Input: part model. Units: mm. Frame: model coordinates. Round coordinates to 2 decimals unless told otherwise and drop trailing zeros. Loops run counter-clockwise (first coordinate to the right, second up) from the corner with the lowest first, then second, coordinate; pieces in that order, holes last.
(1) Cut plane A-A, the plane z = 19.8. Output: boundary loops of the cut face in (x, y).
(2) First-contact query: pin 1 Ø1.6 at (x, z) = (0, 5.8) entering from +Y; pin 2 Ø2.5 at (x, z) = (7, 12.8) entering from -Y; pin 3 Ø3 at (x, z) = (-7, 12.8) entering from +Y; pin 4 Ø5.5 at (x, z) = (0, 5.8) entering from -Y. Flat tips, straight axial feed; report the tip coordinate or a pass-through.
(3) Cut plane B-B, the plane x = 0. Output: boundary loops of the cut face in (y, z).
(4) Line query: line 1 (Z direction, x = 0, y = 1.6); line 2 (Z direction, x = 7, y = 2.3); line 3 (Z direction, x = 0, y = 0.9). Output: solid intervals per line, ascending.
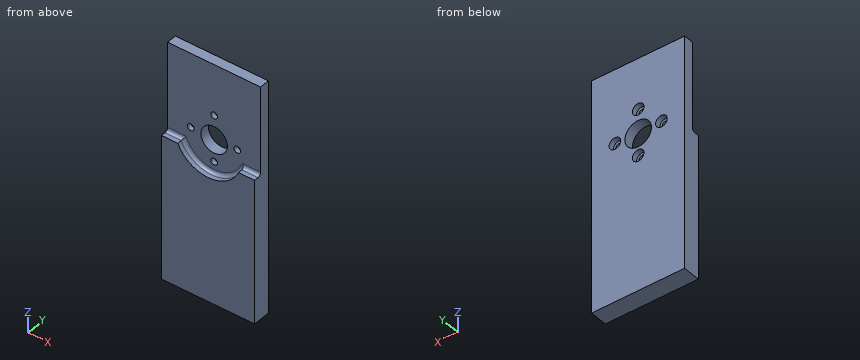
from build123d import *

# Parameters (mm, degrees)
SKETCH1_W           = 28
SKETCH1_H           = 70.4
BOSS_EXTRUDE1_DEPTH = 3
SKETCH4_R           = 1
CUT_EXTRUDE2_DEPTH  = 10
SKETCH5_R           = 4
CUT_EXTRUDE3_DEPTH  = 10
SKETCH10_R          = 1.75
CUT_EXTRUDE9_DEPTH  = 1.6
BOSS_EXTRUDE2_DEPTH = 2.3
FILLET1_R           = 1


with BuildPart() as part:
    # Sketch1 → Boss-Extrude1 (new body)
    with BuildSketch(Plane(origin=(0, 0, 0), x_dir=(1, 0, 0), z_dir=(0, 1, 0))):
        Rectangle(SKETCH1_W, SKETCH1_H)
    extrude(amount=BOSS_EXTRUDE1_DEPTH)

    # Sketch4 → Cut-Extrude2 (cut)
    with BuildSketch(Plane(origin=(0, 3, 0), x_dir=(1, 0, 0), z_dir=(0, 1, 0))):
        with Locations((7, -12.8)):
            Circle(SKETCH4_R)
        with Locations((0, -19.8)):
            Circle(SKETCH4_R)
        with Locations((-7, -12.8)):
            Circle(SKETCH4_R)
        with Locations((0, -5.8)):
            Circle(SKETCH4_R)
    extrude(amount=-CUT_EXTRUDE2_DEPTH, mode=Mode.SUBTRACT)

    # Sketch5 → Cut-Extrude3 (cut)
    with BuildSketch(Plane(origin=(0, 3, 0), x_dir=(1, 0, 0), z_dir=(0, 1, 0))):
        with Locations((0, -12.4)):
            Circle(SKETCH5_R)
    extrude(amount=-CUT_EXTRUDE3_DEPTH, mode=Mode.SUBTRACT)

    # Sketch10 → Cut-Extrude9 (cut)
    with BuildSketch(Plane(origin=(0, 3, 0), x_dir=(1, 0, 0), z_dir=(0, 1, 0))):
        with Locations((0, -19.8)):
            Circle(SKETCH10_R)
        with Locations((-7, -12.8)):
            Circle(SKETCH10_R)
        with Locations((0, -5.8)):
            Circle(SKETCH10_R)
        with Locations((7, -12.8)):
            Circle(SKETCH10_R)
    extrude(amount=-CUT_EXTRUDE9_DEPTH, mode=Mode.SUBTRACT)

    # Sketch11 → Boss-Extrude2 (add)
    with BuildSketch(Plane.XZ):
        with BuildLine():
            Line((9.143433638, 8.350602353), (14, 8.350602353))
            Line((14, 8.350602353), (14, -35.2))
            Line((14, -35.2), (-14, -35.2))
            Line((-14, -35.2), (-14, 8.350602353))
            Line((-14, 8.350602353), (-9.143433638, 8.350602353))
            ThreePointArc((-9.143433638, 8.350602353), (0, 2.4), (9.143433638, 8.350602353))
        make_face()
    extrude(amount=BOSS_EXTRUDE2_DEPTH)

    # Fillet1
    fillet1_edges = [part.edges().sort_by_distance(p)[0] for p in [
        (11.571716819, 0, 8.350602353),
        (0, 0, 2.4),
        (-11.571716819, 0, 8.350602353),
    ]]
    fillet(fillet1_edges, radius=FILLET1_R)


solid = part.part
Reported:
1. outline: (-14, 0) - (-1, 0) - (-1, 1.4) - (-1.75, 1.4) - (-1.75, 3) - (-14, 3) - close; (1, 0) - (14, 0) - (14, 3) - (1.75, 3) - (1.75, 1.4) - (1, 1.4) - close
2. pin 1: passes through
2. pin 2: stops at y = 0
2. pin 3: stops at y = 1.4
2. pin 4: stops at y = -0.06
3. outline: (-2.3, -35.2) - (3, -35.2) - (3, 4.05) - (1.4, 4.05) - (1.4, 4.8) - (0, 4.8) - (0, 3.4) arc R1 cw to (-1, 2.4) - (-2.3, 2.4) - close; (0, 6.8) - (1.4, 6.8) - (1.4, 7.55) - (3, 7.55) - (3, 8.4) - (0, 8.4) - close; (0, 16.4) - (3, 16.4) - (3, 18.05) - (1.4, 18.05) - (1.4, 18.8) - (0, 18.8) - close; (0, 20.8) - (1.4, 20.8) - (1.4, 21.55) - (3, 21.55) - (3, 35.2) - (0, 35.2) - close
4. line 1: z = -35.2 to 4.05, 7.55 to 8.4, 16.4 to 18.05, 21.55 to 35.2
4. line 2: z = -35.2 to 11.05, 14.55 to 35.2
4. line 3: z = -35.2 to 4.8, 6.8 to 8.4, 16.4 to 18.8, 20.8 to 35.2
